```python
from build123d import *

# Parameters (mm, degrees)
SKETCH1_R               = 1.5
BOSS_EXTRUDE1_DEPTH     = 10
SKETCH2_R               = 2
CUT_EXTRUDE1_DEPTH      = 30
SKETCH6_R               = 7.5
BOSS_EXTRUDE3_DEPTH     = 5
CUT_EXTRUDE4_DEPTH      = 26.013853674
CUT_EXTRUDE4_DEPTH_BACK = 26.013853674
SKETCH7_R               = 1.5
SKETCH8_R               = 2
CUT_EXTRUDE5_DEPTH      = 18
SKETCH10_R              = 7.5
CUT_EXTRUDE7_DEPTH      = 9
SKETCH11_W              = 4
SKETCH11_H              = 4
BOSS_EXTRUDE4_DEPTH     = 2.5


with BuildPart() as part:
    # Sketch1 → Boss-Extrude1 (new body)
    with BuildSketch(Plane.XY):
        with BuildLine():
            Line((5.026455026, -10.023549892), (-4.973544974, -10.023549892))
            Line((-4.973544974, -10.023549892), (-4.973544974, 4.386280164))
            ThreePointArc((-4.973544974, 4.386280164), (0.026455026, 17.476450108), (5.026455026, 4.386280164))
            Line((5.026455026, 4.386280164), (5.026455026, -10.023549892))
        make_face()
        with Locations((0.026455026, 9.976450108)):
            Circle(SKETCH1_R, mode=Mode.SUBTRACT)
    extrude(amount=BOSS_EXTRUDE1_DEPTH)

    # Sketch2 → Cut-Extrude1 (cut)
    with BuildSketch(Plane(origin=(0, 0, 0), x_dir=(-1, 0, 0), z_dir=(0, 0, -1))):
        with Locations((-0.026455026, 9.976450108)):
            Circle(SKETCH2_R)
    extrude(amount=-CUT_EXTRUDE1_DEPTH, mode=Mode.SUBTRACT)

    # Sketch6 → Boss-Extrude3 (add, symmetric)
    with BuildSketch(Plane(origin=(2.513227513, 0, 2.513227513), x_dir=(-0.7071067811865477, 0, 0.7071067811865475), z_dir=(-0.7071067811865475, 0, -0.7071067811865477))):
        with Locations((3.516827377, -10.023549892)):
            Circle(SKETCH6_R)
    extrude(amount=BOSS_EXTRUDE3_DEPTH, both=True)

    # Sketch7 → Cut-Extrude4 (cut, two sides: drawn at the far end of the back side and taken through both)
    with BuildSketch(Plane(origin=(-1.022306393, 0, -1.022306393), x_dir=(-0.7071067811865476, 0, 0.7071067811865476), z_dir=(-0.7071067811865476, 0, -0.7071067811865476)).offset(-CUT_EXTRUDE4_DEPTH_BACK)):
        with Locations((3.516827377, -10.023549892)):
            Circle(SKETCH7_R)
    extrude(amount=CUT_EXTRUDE4_DEPTH + CUT_EXTRUDE4_DEPTH_BACK, mode=Mode.SUBTRACT)

    # Sketch8 → Cut-Extrude5 (cut, symmetric)
    with BuildSketch(Plane(origin=(-1.022306393, 0, -1.022306393), x_dir=(-0.7071067811865476, 0, 0.7071067811865476), z_dir=(-0.7071067811865476, 0, -0.7071067811865476))):
        with Locations((3.516827377, -10.023549892)):
            Circle(SKETCH8_R)
    extrude(amount=CUT_EXTRUDE5_DEPTH, both=True, mode=Mode.SUBTRACT)

    # Sketch10 → Cut-Extrude7 (cut)
    with BuildSketch(Plane(origin=(6.048761419, 0, 6.048761419), x_dir=(0.7071067811865476, 0, -0.7071067811865476), z_dir=(0.7071067811865476, 0, 0.7071067811865476))):
        with Locations((-3.516827377, -10.023549892)):
            Circle(SKETCH10_R)
    cut_extrude7 = extrude(amount=CUT_EXTRUDE7_DEPTH, mode=Mode.SUBTRACT)

    # Mirror1: Cut-Extrude7 across plane
    add(cut_extrude7.mirror(Plane(origin=(2.513227513, 0, 2.513227513), x_dir=(-0.7071067811865478, 0, 0.7071067811865472), z_dir=(-0.7071067811865475, 0, -0.7071067811865477))), mode=Mode.SUBTRACT)

    # Sketch11 → Boss-Extrude4 (add, symmetric)
    with BuildSketch(Plane(origin=(0, -17.5, 0), x_dir=(1, 0, 0), z_dir=(0, 1, 0))):
        with Locations((0.026455026, -5)):
            Rectangle(SKETCH11_W, SKETCH11_H)
    extrude(amount=BOSS_EXTRUDE4_DEPTH, both=True)


solid = part.part
```
Geometry: final body of the model. Coordinates: model frame, mm. A direction names the side the tool comes from. Round coordinates to 2 decimals unless told otherwise and drop trailing zeros. Write each loop counter-clockwise with the first axis right and the second up, starting at its lowest first coordinate (ties: lowest second). Pieces come first, ordered by that corner, then holes. Notation, with made-up numbers: M 10.25,55 L 28.25,55 A25 cw 28.25,69 Z; hole C 43,12.25 d3. An arc over 180 degrees is marked long. Answer in a Markdown table with one row per item. Add a question column.
(1) Cut plane B-B, the plane y = 2. Return the cut outline in (x, z).
(2) Ray query, L1, parallel to Z at x = 0, y = 4; L2, parallel to Y at x = -1, z = 1; L3, parallel to X at y = 11, z = 0.25. Return the intervals inside material, ascending.
(3) Contact query for flat-ended pins moving along their axis: pin 1 (3 mm diameter, centred on x = 6.5, z = 3, fed in from -Y); pin 2 (4.5 mm diameter, centred on x = 3, y = -0.5, fed in from -Z); pin 3 (6 mm diameter, centred on y = 11.5, z = 2.5, fed in from +X). Output: stop coordinate, or through.
(4) Draft query along Z for faces 3 (the face through (0, -19, 7)), 4 (the face through (0, -19, 3)), 5 (the face through (5.026, 0, 5)), 6 (the face through (0.16, -8.04, 4.77)). Return one class per face: pulls with the +Z half, pulls with the -Z half, needs draft (parallel to the pull), parting line crosses it, or undercut.
(5) Cut plane A-A, the plane y = -9.5. Return the cut outline in (x, z).
(6) Reachability of faces 1 (the face through (-0.227, 17.472, 4.93)), 2 (the face through (-4.974, 0, 5)) from +Z, -Z, +X, -X, +Y, -Y: full face, straight path, thin tool, end or side. Return the list, or none.
(7) Cut plane C-C, the plane x = 0.25. Give the number of separate pieces and of enclosed holes in the cut face, then the cut area to 3 significant figures.
Established:
| question | item | result |
|---|---|---|
| 1 | outline | M -4.97,0 L 5.03,0 L 5.03,10 L -4.97,10 Z |
| 2 | L1 | 0 to 10 |
| 2 | L2 | -17.22 to 8.26, 11.69 to 17.41 |
| 2 | L3 | -7.4 to -1.69, 1.74 to 7.46 |
| 3 | pin 1 | y = -16.03 |
| 3 | pin 2 | z = 0 |
| 3 | pin 3 | x = 7.53 |
| 4 | face 3 | pulls with the +Z half |
| 4 | face 4 | pulls with the -Z half |
| 4 | face 5 | needs draft |
| 4 | face 6 | undercut |
| 5 | outline | M -8.8,6.75 L -4.87,2.83 L 2.2,9.9 L -1.73,13.83 Z; M -2.14,0.1 L 1.78,-3.83 L 8.85,3.25 L 4.93,7.17 Z |
| 6 | face 1 | +Z, -Z |
| 6 | face 2 | +Z, -X |
| 7 | separate pieces | 2 |
| 7 | enclosed holes | 1 |
| 7 | area | 350 mm² |
